```python
from build123d import *

# Parameters (mm, degrees)
SKETCH1_R                                         = 76.2
BOSS_EXTRUDE1_DEPTH                               = 6.35
SKETCH2_R                                         = 6.35
BOSS_EXTRUDE2_DEPTH                               = 20.32
CIRPATTERN1_COUNT                                 = 3
F_5_8_0_625_DIAMETER_HOLE1_D                      = 15.875
SKETCH11_R                                        = 9.525
BOSS_EXTRUDE3_DEPTH                               = 3.175
CIRPATTERN5_COUNT                                 = 3
CUT_EXTRUDE3_REACH                                = 111.662
SKETCH12_R                                        = 22.86
SKETCH13_W                                        = 1.905
SKETCH13_H                                        = 1.27
CIRPATTERN6_COUNT                                 = 3
CHAMFER1_SIZE                                     = 1.27
CUT_EXTRUDE4_REACH                                = 111.662
SKETCH14_R                                        = 15.875
CIRPATTERN7_COUNT                                 = 3
CHAMFER2_SIZE                                     = 1.27
SKETCH15_W                                        = 38.1
SKETCH15_H                                        = 64.057059502
BOSS_EXTRUDE4_DEPTH                               = 6.35
FILLET1_RADIUS                                    = 19.05
FILLET1_LENGTH                                    = 6.35
BOSS_EXTRUDE5_DEPTH                               = 6.35
F_10_0_5_DIAMETER_HOLE1_D                         = 12.7
CSK_FOR_8_FLAT_HEAD_MACHINE_SCREW_100_D           = 4.4958
CSK_FOR_8_FLAT_HEAD_MACHINE_SCREW_100_CSINK_D     = 8.4328
CSK_FOR_8_FLAT_HEAD_MACHINE_SCREW_100_CSINK_ANGLE = 100
MIRROR3_COPY_1_DEPTH                              = 6.35
FILLET1_OF_MIRROR3_2_RADIUS                       = 19.05
FILLET1_OF_MIRROR3_2_LENGTH                       = 6.35
CHAMFER3_SIZE                                     = 1.27


with BuildPart() as part:
    # Sketch1 → Boss-Extrude1 (new body)
    with BuildSketch(Plane.XY):
        Circle(SKETCH1_R)
    extrude(amount=-BOSS_EXTRUDE1_DEPTH)

    # Sketch2 → Boss-Extrude2 (add)
    with BuildSketch(Plane.XY):
        with Locations((0, 49.7078)):
            Circle(SKETCH2_R)
    boss_extrude2 = extrude(amount=BOSS_EXTRUDE2_DEPTH)

    # CirPattern1: Boss-Extrude2 ×3 about axis
    cirpattern1_axis = Axis((0, 0, 0), (0, 0, 1))
    for i in range(1, CIRPATTERN1_COUNT):
        add(boss_extrude2.rotate(cirpattern1_axis, i * 360 / CIRPATTERN1_COUNT))

    # 5/8 (0.625) Diameter Hole1 (through all)
    with Locations(Plane.XY):
        with Locations((0, 0)):
            Hole(F_5_8_0_625_DIAMETER_HOLE1_D / 2)

    # Sketch11 → Boss-Extrude3 (add)
    with BuildSketch(Plane.XY):
        with Locations((0, 49.7078)):
            Circle(SKETCH11_R)
    boss_extrude3 = extrude(amount=BOSS_EXTRUDE3_DEPTH)

    # CirPattern5: Boss-Extrude3 ×3 about axis
    cirpattern5_axis = Axis((0, 0, 0), (0, 0, 1))
    for i in range(1, CIRPATTERN5_COUNT):
        add(boss_extrude3.rotate(cirpattern5_axis, i * 360 / CIRPATTERN5_COUNT))

    # Sketch12 → Cut-Extrude3 (cut, up to next)
    with BuildSketch(Plane.XY, mode=Mode.PRIVATE) as cut_extrude3_sk1:
        Circle(SKETCH12_R)
    cut_extrude3_tool1 = extrude(cut_extrude3_sk1.sketch, amount=-CUT_EXTRUDE3_REACH, mode=Mode.PRIVATE) & part.part
    add(cut_extrude3_tool1.solids().sort_by_distance((0, 0, 0))[0], mode=Mode.SUBTRACT)

    # Sketch13 → Cut-Revolve1 (revolve, cut)
    with BuildSketch(Plane(origin=(0, 0, 0), x_dir=(0, 0, -1), z_dir=(1, 0, 0)), mode=Mode.PRIVATE) as cut_revolve1_sk:
        with Locations((-18.0975, 56.0578)):
            Rectangle(SKETCH13_W, SKETCH13_H)
    cut_revolve1 = revolve(cut_revolve1_sk.sketch.rotate(Axis((0, 49.7078, 20.32), (0, 0, 1)), 90), axis=Axis((0, 49.7078, 20.32), (0, 0, 1)), mode=Mode.SUBTRACT)

    # CirPattern6: Cut-Revolve1 ×3 about axis
    cirpattern6_axis = Axis((0, 0, 0), (0, 0, 1))
    for i in range(1, CIRPATTERN6_COUNT):
        add(cut_revolve1.rotate(cirpattern6_axis, i * 360 / CIRPATTERN6_COUNT), mode=Mode.SUBTRACT)

    # Chamfer1
    chamfer1_edges = [part.edges().sort_by_distance(p)[0] for p in [
        (-76.2, 0, 0),
        (-9.525, 49.7078, 0),
        (-38.285717566, -33.102791971, 0),
        (47.810717566, -16.605008029, 0),
        (-22.86, 0, -6.35),
        (-22.86, 0, 0),
        (-76.2, 0, -6.35),
    ]]
    chamfer(chamfer1_edges, length=CHAMFER1_SIZE)

    # Sketch14 → Cut-Extrude4 (cut, up to next)
    with BuildSketch(Plane.XY, mode=Mode.PRIVATE) as cut_extrude4_sk1:
        with Locations((42.894238249, 24.765)):
            Circle(SKETCH14_R)
    cut_extrude4_tool1 = extrude(cut_extrude4_sk1.sketch, amount=-CUT_EXTRUDE4_REACH, mode=Mode.PRIVATE) & part.part
    cut_extrude4 = cut_extrude4_tool1.solids().sort_by_distance((42.894238, 24.765, 0))[0]
    add(cut_extrude4, mode=Mode.SUBTRACT)

    # CirPattern7: Cut-Extrude4 ×3 about axis
    cirpattern7_axis = Axis((0, 0, 0), (0, 0, 1))
    for i in range(1, CIRPATTERN7_COUNT):
        add(cut_extrude4.rotate(cirpattern7_axis, i * 360 / CIRPATTERN7_COUNT), mode=Mode.SUBTRACT)

    # Chamfer2
    chamfer2_edges = [part.edges().sort_by_distance(p)[0] for p in [
        (7.9375, -35.781846715, -6.35),
        (27.019238249, 24.765, 0),
        (27.019238249, 24.765, -6.35),
        (-34.956738249, 11.016846715, 0),
        (-34.956738249, 11.016846715, -6.35),
        (7.9375, -35.781846715, 0),
    ]]
    chamfer(chamfer2_edges, length=CHAMFER2_SIZE)

    # Sketch15 → Boss-Extrude4 (add)
    with BuildSketch(Plane.XY):
        with Locations((0, 104.496470249)):
            Rectangle(SKETCH15_W, SKETCH15_H)
    boss_extrude4 = extrude(amount=-BOSS_EXTRUDE4_DEPTH)

    # Fillet1: full round fillet: the end face becomes a half cylinder, R = half its width
    fillet1_face = Plane((0, 136.525, -3.175), x_dir=(0, 0, 1), z_dir=(0, 1, 0))  # on the end face: x along it, z out of the body
    fillet1_slab = fillet1_face.offset(-FILLET1_RADIUS / 2) * Box(FILLET1_LENGTH, 2 * FILLET1_RADIUS, FILLET1_RADIUS, mode=Mode.PRIVATE)  # the body's end, R deep
    fillet1_round = Plane((0, 117.475, -3.175), x_dir=(0, 1, 0), z_dir=(0, 0, 1)) * Cylinder(FILLET1_RADIUS, FILLET1_LENGTH, mode=Mode.PRIVATE)  # its axis R under the face
    add(fillet1_slab - fillet1_round, mode=Mode.SUBTRACT)

    # Sketch16 → Boss-Extrude5 (add)
    with BuildSketch(Plane.XY):
        with BuildLine():
            Line((-19.05, 85.910595388), (-19.05, 72.467940498))
            ThreePointArc((-19.05, 72.467940498), (-24.793169644, 70.709289623), (-30.377027027, 68.496285512))
            ThreePointArc((-30.377027027, 68.496285512), (-22.130887076, 75.523587521), (-19.05, 85.910595388))
        make_face()
    boss_extrude5 = extrude(amount=-BOSS_EXTRUDE5_DEPTH)

    # Mirror1: Boss-Extrude5 across plane
    add(boss_extrude5.mirror(Plane(origin=(0, 0, 0), x_dir=(0, 0, 1), z_dir=(1, 0, 0))))

    # #10 (0.5) Diameter Hole1 (through all)
    with Locations(Plane.XY):
        with Locations((0, 117.475)):
            f_10_0_5_diameter_hole1 = Hole(F_10_0_5_DIAMETER_HOLE1_D / 2)

    # CSK for #8 Flat Head Machine Screw (100)1 (through all)
    with Locations(Plane(origin=(0, 0, -6.35), x_dir=(-1, 0, 0), z_dir=(0, 0, -1))):
        with Locations((12.7, 97.602206046), (-12.7, 97.602206046)):
            csk_for_8_flat_head_machine_screw_100 = CounterSinkHole(CSK_FOR_8_FLAT_HEAD_MACHINE_SCREW_100_D / 2, CSK_FOR_8_FLAT_HEAD_MACHINE_SCREW_100_CSINK_D / 2, counter_sink_angle=CSK_FOR_8_FLAT_HEAD_MACHINE_SCREW_100_CSINK_ANGLE)

    # Mirror3: Boss-Extrude4, Boss-Extrude5, #10 (0.5) Diameter Hole1, CSK for #8 Flat Head Machine Screw (100)1 across plane
    add(boss_extrude4.mirror(Plane.ZX))
    add(boss_extrude5.mirror(Plane.ZX))
    add(f_10_0_5_diameter_hole1.mirror(Plane.ZX), mode=Mode.SUBTRACT)
    add(csk_for_8_flat_head_machine_screw_100.mirror(Plane.ZX), mode=Mode.SUBTRACT)

    # Mirror3 copy 1 sketch → Mirror3 copy 1 (add)
    with BuildSketch(Plane(origin=(0, 0, 0), x_dir=(-1, 0, 0), z_dir=(0, 0, 1))):
        with BuildLine():
            Line((-19.05, 85.910595388), (-19.05, 72.467940498))
            ThreePointArc((-19.05, 72.467940498), (-24.793169644, 70.709289623), (-30.377027027, 68.496285512))
            ThreePointArc((-30.377027027, 68.496285512), (-22.130887076, 75.523587521), (-19.05, 85.910595388))
        make_face()
    extrude(amount=-MIRROR3_COPY_1_DEPTH)

    # Fillet1 of Mirror3 2: full round fillet: the end face becomes a half cylinder, R = half its width
    fillet1_of_mirror3_2_face = Plane((0, -136.525, -3.175), x_dir=(0, 0, 1), z_dir=(0, -1, 0))  # on the end face: x along it, z out of the body
    fillet1_of_mirror3_2_slab = fillet1_of_mirror3_2_face.offset(-FILLET1_OF_MIRROR3_2_RADIUS / 2) * Box(FILLET1_OF_MIRROR3_2_LENGTH, 2 * FILLET1_OF_MIRROR3_2_RADIUS, FILLET1_OF_MIRROR3_2_RADIUS, mode=Mode.PRIVATE)  # the body's end, R deep
    fillet1_of_mirror3_2_round = Plane((0, -117.475, -3.175), x_dir=(0, -1, 0), z_dir=(0, 0, 1)) * Cylinder(FILLET1_OF_MIRROR3_2_RADIUS, FILLET1_OF_MIRROR3_2_LENGTH, mode=Mode.PRIVATE)  # its axis R under the face
    add(fillet1_of_mirror3_2_slab - fillet1_of_mirror3_2_round, mode=Mode.SUBTRACT)

    # Chamfer3
    chamfer3_edges = [part.edges().sort_by_distance(p)[0] for p in [
        (-19.05, 101.692797694, 0),
        (-19.05, 101.692797694, -6.35),
        (0, 136.525, 0),
        (0, 136.525, -6.35),
        (-22.130887076, 75.523587521, -6.35),
        (-22.130887076, 75.523587521, 0),
        (19.05, 101.692797694, -6.35),
        (19.05, 101.692797694, 0),
        (22.130887076, 75.523587521, 0),
        (22.130887076, 75.523587521, -6.35),
        (-19.05, -101.692797694, -6.35),
        (-19.05, -101.692797694, 0),
        (0, -136.525, -6.35),
        (0, -136.525, 0),
        (-22.130887076, -75.523587521, 0),
        (-22.130887076, -75.523587521, -6.35),
        (19.05, -101.692797694, 0),
        (19.05, -101.692797694, -6.35),
        (22.130887076, -75.523587521, -6.35),
        (22.130887076, -75.523587521, 0),
    ]]
    chamfer(chamfer3_edges, length=CHAMFER3_SIZE)


solid = part.part
```
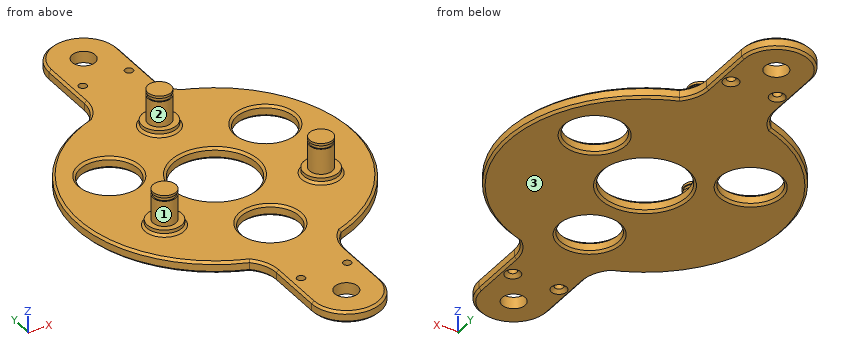
Can you work these out from the model? Positions are in its coordinate system, mm. Face numbers are marked on the shaded views. Coordinates: 2 decimals unless noted, no trailing zeros. Loops run counter-clockwise (first coordinate to the right, second up) from the corner with the lowest first, then second, coordinate; pieces in that order, holes last.
1) Imagine slicing it at C-C on z = 8.5. List the corners of the cut face in (x, y) for me, plus the area to 3 significant figures.
2) Imagine slicing it at B-B on x = 0. State how many separate pieces and enclosed holes the cut face has, plus the area to 3 significant figures.
3) I need wall thicknesses on probe 1 along Y at (x, z) = (0, -5) (3 decimals); probe 2 along Y at (x, z) = (1, -0.75); probe 3 along X at (y, z) = (52.5, 15.5). Which ranges of each line are inside material? Lowest first, please.
4) Imagine slicing it at A-A on y = 0. List the corners of the cut face in (x, z) for me, plus the area to 3 significant figures.
5) For pin 1 (8 mm diameter, centred on y = -62.5, z = 3, fed in from -X); pin 2 (5 mm diameter, centred on x = -32.5, z = 1, fed in from +Y); pin 3 (10 mm diameter, centred on x = 0, y = 117.475, fed in from +Z); pin 4 (12 mm diameter, centred on x = 33.5, z = 11, fed in from -Y), each with a flat end and sliding along its axis, tell me the tip position at first contact or that it passes through.
6) Thinking about a two-plate mould opening in X: for the marked faces 1, 2 and 3, which applies, pulls with the +X half, pulls with the -X half, needs draft (parallel to the pull), parting line crosses it, or undercut?
Completed:
1. outline: circle Ø12.7 at (-43.05, -24.85); circle Ø12.7 at (0, 49.71); circle Ø12.7 at (43.05, -24.85)
1. area: 380 mm2
2. separate pieces: 5
2. enclosed holes: 0
2. area: 1,350 mm2
3. probe 1: y = -136.525 to -123.825, -111.125 to -65.405, -33.655 to -22.86, 22.86 to 111.125, 123.825 to 136.525
3. probe 2: y = -135.98 to -123.75, -111.2 to -65.89, -33.17 to -23.36, 23.36 to 111.2, 123.75 to 135.98
3. probe 3: x = -5.7 to 5.7
4. outline: (-76.2, -5.08) - (-74.93, -6.35) - (-24.13, -6.35) - (-22.86, -5.08) - (-22.86, -1.27) - (-24.13, 0) - (-74.93, 0) - (-76.2, -1.27) - close; (22.86, -5.08) - (24.13, -6.35) - (74.93, -6.35) - (76.2, -5.08) - (76.2, -1.27) - (74.93, 0) - (24.13, 0) - (22.86, -1.27) - close
4. area: 671 mm2
5. pin 1: stops at x = -45.09
5. pin 2: stops at y = 69.41
5. pin 3: passes through
5. pin 4: stops at y = -30.12
6. face 1: undercut
6. face 2: parting line crosses it
6. face 3: needs draft
